CAD build for the part. Positions are in the model's coordinates, mm. Round coordinates to 2 decimals unless told otherwise and drop trailing zeros. Write each loop counter-clockwise with the first axis right and the second up, starting at its lowest first coordinate (ties: lowest second). Pieces come first, ordered by that corner, then holes. Notation, with made-up numbers: (23.5, -19.5) -> (29.5, -19.5) arc R16 cw to (29.5, 11.5) -> close; hole circle Ø5 at (-34.75, 59.5). An arc over 180 degrees is marked (long way). Put each result on its own line as item: value. Start each with the question number.
1. Flat gauge pin, fed straight in: P1, Ø1.2, axis at x = 47.04, y = -0.04, coming from the +Z side. Where does the tip first touch, or does it go through?
2. Saw through at A-A on x = 0. List the corners of the cut face in (y, z).
3. Pull direction X, two halves, no side cores. Call faces 1 (the cylindrical face through (-2.5, -0.09, 0.69)), 2 (the flat face through (23, 0, 0)), 3 (the cylindrical face through (49.536, 0.051, 0.69)): pulls with the +X half, pulls with the -X half, needs draft (parallel to the pull), parting line crosses it, or undercut.
4. Saw through at C-C on y = -1.9. List the corners of the cut face in (x, z), and give its area (3 significant figures).
5. Saw through at B-B on z = 0.3. State how many separate pieces and enclosed holes the cut face has, and give its area (3 significant figures).
6. Saw through at D-D on x = 12. List the corners of the cut face in (y, z), and give its area (3 significant figures).
7. Drill centre lines: line 1 (X direction, y = 0, z = 1); line 2 (Y direction, x = 0, z = 0.65); line 3 (X direction, y = -0.7, z = 0.4). Where is each one in solid material? Low to high. Write a range as from..to.
Autodesk Inventor part; units mm, degrees
ref_plane "YZ Plane" through (0, 0, 0) normal (1, 0, 0) x (0, 1, 0)
ref_plane "XZ Plane" through (0, 0, 0) normal (0, 1, 0) x (-1, 0, 0)
ref_plane "XY Plane" through (0, 0, 0) normal (0, 0, 1) x (1, 0, 0)
sketch "Sketch1" plane through (0, 0, 0) normal (0, 0, 1) x (1, 0, 0)
  circle A0 centre (0, 0) radius 1
  circle A1 centre (47.0377, -0.0423) radius 1
  arc A2 (2.2923, 0.9976) -> (2.2904, -1.0021) centre (0, 0) ccw
  arc A3 (44.7455, -1.0402) -> (44.7473, 0.9598) centre (47.0377, -0.0423) ccw
  line L0 (0, -2) -> (0, 1)
  line L1 (48.4179, 2.0423) -> (48.671, 2.0423)
  line L2 (48.671, -1.9577) -> (48.6442, -1.9577)
  line L3 (48.671, 2.0423) -> (48.671, 1.8505)
  line L4 (48.671, -1.935) -> (48.671, -1.9577)
  line L5 (0, 1) -> (0.0018, 1)
  line L6 (2.2923, 0.9976) -> (44.7473, 0.9598)
  line L7 (47.0404, -1.0422) -> (47.0368, -1.0423)
  line L8 (44.7455, -1.0402) -> (2.2904, -1.0021)
  dimension "d0" = 2
  dimension "d1" = 2
  dimension "d2" = 5
  dimension "d3" = 5
  dimension "d5" = 4
extrude "Extrusion1" add sketch "Sketch1" along normal blind 1.4 contours L6 A3 L8 A2
sketch "Sketch2" plane through (0, 0, 0) normal (0, 0, -1) x (-1, 0, 0)
  point P0 (0, 0)
properties part number "Restrain_Pin_1"
Return value:
1. P1: passes through
2. outline: (-2.5, 0) -> (-1, 0) -> (-1, 1.4) -> (-2.5, 1.4) -> close; (1, 0) -> (2.5, 0) -> (2.5, 1.4) -> (1, 1.4) -> close
3. face 1: undercut
3. face 2: needs draft
3. face 3: undercut
4. outline: (-1.62, 0) -> (1.62, 0) -> (1.62, 1.4) -> (-1.62, 1.4) -> close; (45.36, 0) -> (48.71, 0) -> (48.71, 1.4) -> (45.36, 1.4) -> close
4. area: 9.23 mm^2
5. separate pieces: 1
5. enclosed holes: 2
5. area: 117 mm^2
6. outline: (-1.01, 0) -> (0.99, 0) -> (0.99, 1.4) -> (-1.01, 1.4) -> close
6. area: 2.80 mm^2
7. line 1: x = -2.5..-1, 1..46.04, 48.04..49.54
7. line 2: y = -2.5..-1, 1..2.5
7. line 3: x = -2.4..-0.71, 0.71..46.28, 47.79..49.45
